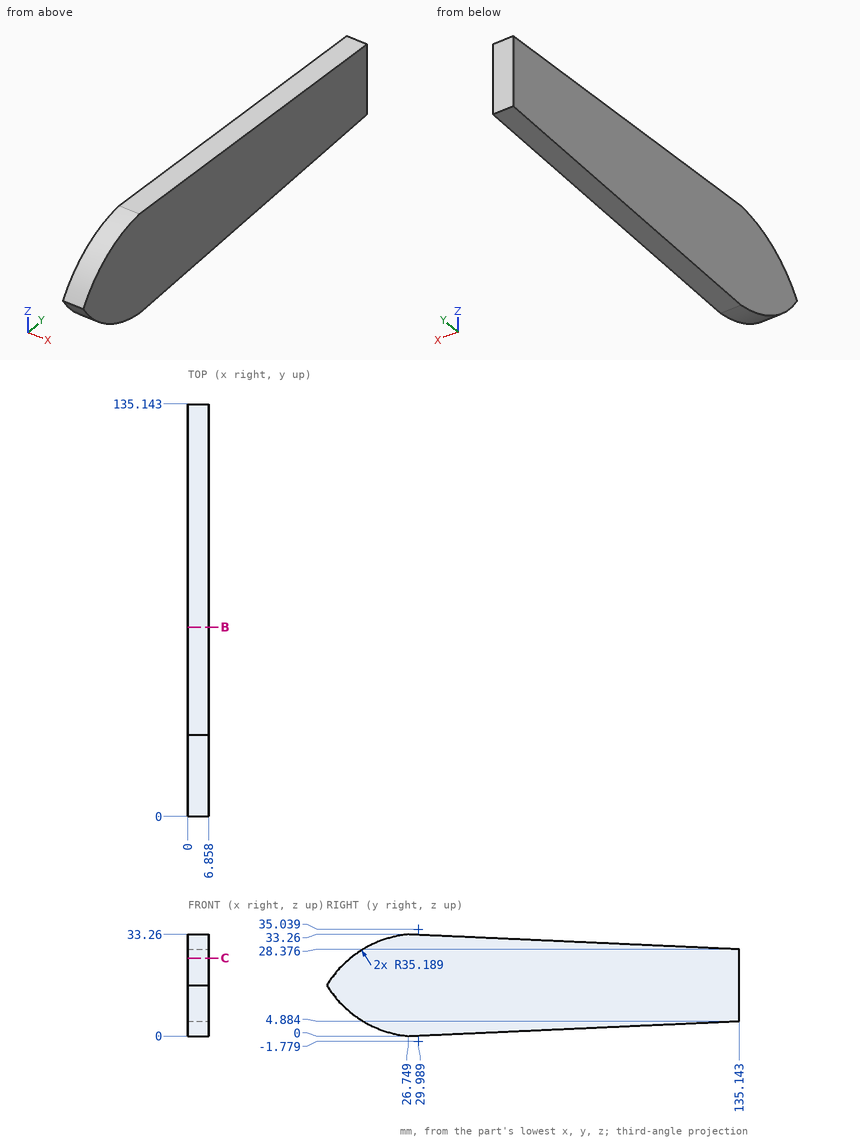
Can you work these out from the drawing? Everything is in mm from the part's minimum corner. Give positions to 0.01 mm unless a question says otherwise; leave off trailing zeros. Order: outer loops, then holes, each group sorted by start corner. A loop starts at its lowest first (then second) coordinate and runs counter-clockwise, first axis right, second up. Notation, with made-up numbers: M 3,-29 L 36,-29 A9 cw 36,-17 Z; hole C -10.5,49.25 d2. An arc over 180 degrees is marked long. Write item = value, one per line. Start each with the question number.
Q1. I need wall thicknesses on probe 1 along Z at (x, y) = (3.75, 27); probe 2 along Y at (x, z) = (1.25, 5) (1 decimal); probe 3 along Y at (x, z) = (5.5, 12). Which ranges of each line are inside material? Lowest first, please. Write a range as [from, to].
Q2. Suppose I cut it at C-C (z = 25.5). Write out the boundary of the cut face in (x, y).
Q3. Suppose I cut it at B-B (y = 62). Write out the boundary of the cut face in (x, z).
Q4. Will these pins go through, and if not, where does the flat tip stop? pin 1 Ø3 at (x, z) = (1, 18.5) entering from -Y; pin 2 Ø1.5 at (x, z) = (5, 22.5) entering from -Y (1 decimal); pin 3 Ø2 at (x, y) = (2.5, 70.5) entering from -Z.
Check result:
q1.probe_1 = [0.01, 33.25]
q1.probe_2 = [11.7, 135.1]
q1.probe_3 = [3.39, 135.14]
q2.outline = M 0,7.76 L 6.86,7.76 L 6.86,135.14 L 0,135.14 Z
q3.outline = M 0,1.59 L 6.86,1.59 L 6.86,31.67 L 0,31.67 Z
q4.pin_1 = 0.23
q4.pin_2 = 3.8
q4.pin_3 = 1.93
